Can you work these out from the drawing? Everything is in mm from the part's minimum corner. A direction names the side the tool comes from. Give positions to 0.01 mm unless a question says otherwise; leave off trailing zeros. Write each loop counter-clockwise with the first axis right and the second up, starting at its lowest first coordinate (ties: lowest second). Pieces come first, ordered by that corner, then holes. Notation, with made-up numbers: (16.25, 37.5) -> (45.25, 37.5) arc R20 ccw to (45.25, 76.5) -> close; hole circle Ø7 at (34.5, 43.5). An arc over 180 degrees is marked (long way). Return JSON: item names as keys, results as strings.
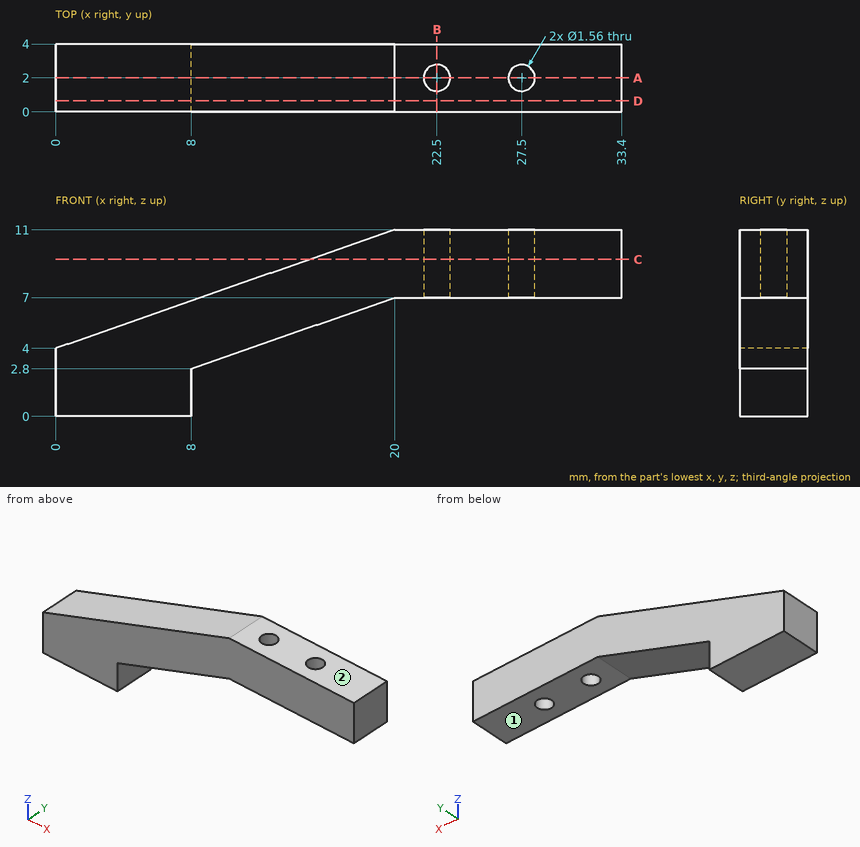
1. Which directions (+Z, -Z, +X, -X, +Y, -Y) give clear straight access to the entire face, cutting with the end or side of a thin tool? Please do the marked faces 1 and 2.
Taken from the geometry:
{"face 1": "-Z, +X, +Y, -Y", "face 2": "+Z, +X, -X, +Y, -Y"}
2. Suppose I cut it at D-D, the plane y = 0.65. List the corners of the cut face in (x, z) for me.
Taken from the geometry:
{"outline": "(0, 0) -> (8, 0) -> (8, 2.8) -> (20, 7) -> (33.4, 7) -> (33.4, 11) -> (20, 11) -> (0, 4) -> close"}
3. Suppose I cut it at A-A, the plane y = 2. List the corners of the cut face in (x, z) for me.
Taken from the geometry:
{"outline": "(0, 0) -> (8, 0) -> (8, 2.8) -> (20, 7) -> (21.72, 7) -> (21.72, 11) -> (20, 11) -> (0, 4) -> close; (23.28, 7) -> (26.72, 7) -> (26.72, 11) -> (23.28, 11) -> close; (28.28, 7) -> (33.4, 7) -> (33.4, 11) -> (28.28, 11) -> close"}
4. If I drill on line 1 (Y direction, x = 27.5, z = 9.25); line 2 (X direction, y = 2.1, z = 2.5); line 3 (Z direction, x = 26, y = 0.95), over which ranges is the centre line in solid material (lowest first)? Write a range as [from, to].
Taken from the geometry:
{"line 1": "y = [0, 1.22], [2.78, 4]", "line 2": "x = [0, 8]", "line 3": "z = [7, 11]"}
5. Suppose I cut it at C-C, the plane z = 9.25. List the corners of the cut face in (x, y) for me.
Taken from the geometry:
{"outline": "(15, 0) -> (33.4, 0) -> (33.4, 4) -> (15, 4) -> close; hole circle Ø1.56 at (22.5, 2); hole circle Ø1.56 at (27.5, 2)"}
6. Suppose I cut it at B-B, the plane x = 22.5. List the corners of the cut face in (y, z) for me, and give its area (3 significant figures).
Taken from the geometry:
{"outline": "(0, 7) -> (1.22, 7) -> (1.22, 11) -> (0, 11) -> close; (2.78, 7) -> (4, 7) -> (4, 11) -> (2.78, 11) -> close", "area": "9.76 mm²"}
7. For pin 1 Ø2 at (x, y) = (28, 2.5) entering from +Z; pin 2 Ø2 at (x, y) = (26.5, 0.5) entering from -Z; pin 3 Ø1.5 at (x, y) = (13, 3) entering from +Z, each with a flat end and sliding along its axis, tell me the tip position at first contact or that it passes through.
Taken from the geometry:
{"pin 1": "stops at z = 11", "pin 2": "stops at z = 7", "pin 3": "stops at z = 8.81"}
